For this review, use the dimensioned drawing (mm, ordinates from the lowest corner) and the shaded views. A direction names the side the tool comes from. Give positions to 0.01 mm unless a question says otherwise; leave off trailing zeros. Loops run counter-clockwise (first coordinate to the right, second up) from the corner with the lowest first, then second, coordinate; pieces in that order, holes last. Notation, with made-up numbers: M 71.25,8 L 104.25,8 A14 ccw 104.25,24 Z; hole C -6,13.25 d6. An arc over 180 degrees is marked long. Use a Markdown table: item, result. Add a question column.
(1) For the marked faces 4 and 5, list the 3-axis set-ups (+Z, -Z, +X, -X, +Y, -Y) from which the entire face can be reached by the end or side of a thin tool; tool diameter is ignored.
(2) Draft analysis for pull direction Z (two halves, no side actions). For the marked faces 1, 2 and 3, state which applies: pulls with the +Z half, pulls with the -Z half, needs draft (parallel to the pull), parting line crosses it, or undercut.
(3) Add section B-B, the plane z = 41.1. Give the boundary of the cut face in (x, y), then the cut area to 3 significant figures.
(4) Add section A-A, the plane x = 47. Give the boundary of the cut face in (y, z) (1 decimal).
(5) Insertion check: pin 1 Ø6 at (x, y) = (50.8, 63.5) entering from -Z; pin 2 Ø6 at (x, z) = (29, 6.5) entering from -Y; pin 3 Ø3 at (y, z) = (10.5, 43.5) entering from +X; pin 4 Ø1.9 at (x, z) = (2.5, 29) entering from +Y. Each pin has a flat end and moves straight along its axis. Give the tip position at first contact, or say it passes through.
(6) For probe 1 along X at (y, z) = (63.5, 2.35); probe 2 along Y at (x, z) = (2.25, 15.7); probe 3 along Z at (x, y) = (32, 55), list the stretches that pass through material, from the lowest coordinate up.
(7) Add section C-C, the plane y = 25.4. Give the boundary of the cut face in (x, z) (1 decimal).
(8) Add section D-D, the plane x = 38.1. Give the boundary of the cut face in (y, z) (1 decimal).
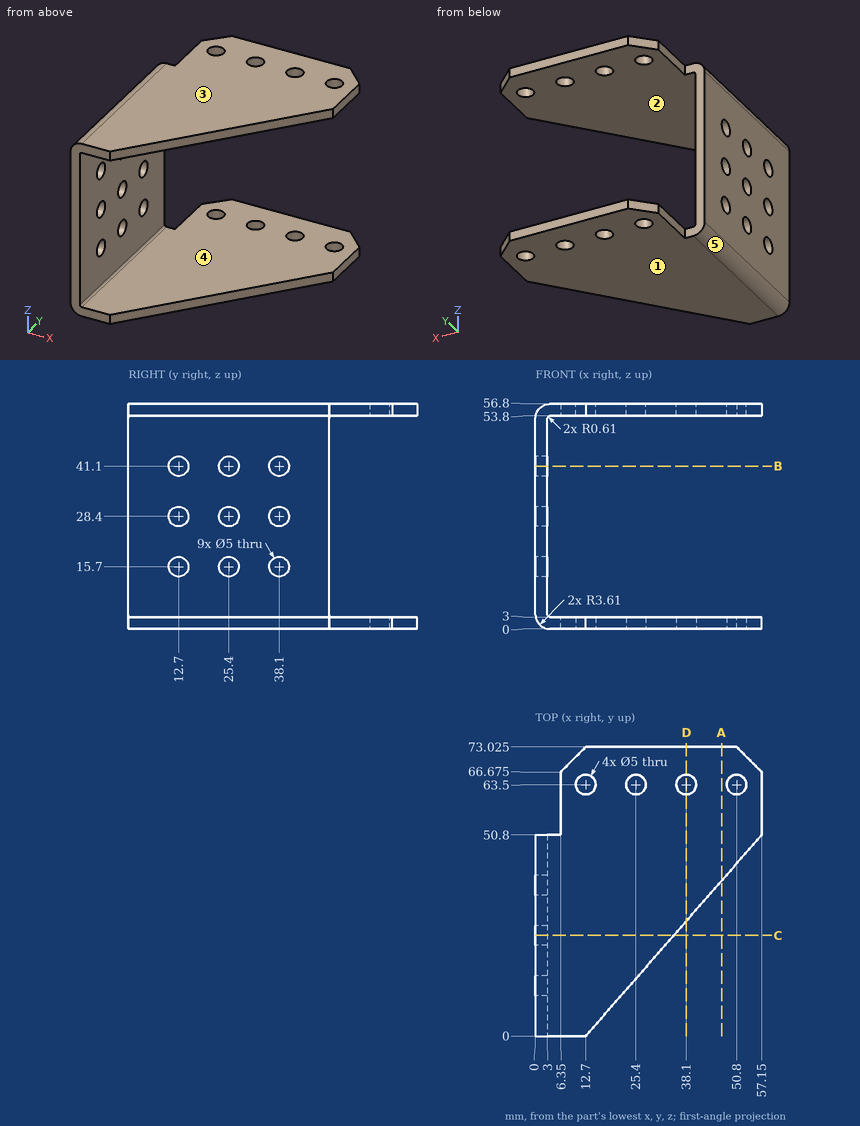
Established:
| question | item | result |
|---|---|---|
| 1 | face 4 | +X, +Y, -Y |
| 1 | face 5 | -Z, -X, +Y, -Y |
| 2 | face 1 | pulls with the -Z half |
| 2 | face 2 | undercut |
| 2 | face 3 | pulls with the +Z half |
| 3 | outline | M 0,0 L 3,0 L 3,10.2 L 0,10.2 Z; M 0,15.2 L 3,15.2 L 3,22.9 L 0,22.9 Z; M 0,27.9 L 3,27.9 L 3,35.6 L 0,35.6 Z; M 0,40.6 L 3,40.6 L 3,50.8 L 0,50.8 Z |
| 3 | area | 107 mm^2 |
| 4 | outline | M 39.2,0 L 73,0 L 73,3 L 39.2,3 Z; M 39.2,53.8 L 73,53.8 L 73,56.8 L 39.2,56.8 Z |
| 5 | pin 1 | z = 0 |
| 5 | pin 2 | through |
| 5 | pin 3 | x = 3 |
| 5 | pin 4 | y = 50.8 |
| 6 | probe 1 | 6.35 to 10.2, 15.2 to 22.9, 27.9 to 35.6, 40.6 to 48.3, 53.3 to 57.15 |
| 6 | probe 2 | 0 to 10.2, 15.2 to 22.9, 27.9 to 35.6, 40.6 to 50.8 |
| 6 | probe 3 | 0 to 3, 53.8 to 56.8 |
| 7 | outline | M 0,3.6 A3.6 ccw 3.6,0 L 34.9,0 L 34.9,3 L 3.6,3 A0.6 cw 3,3.6 L 3,13.2 L 0,13.2 Z; M 0,18.2 L 3,18.2 L 3,25.9 L 0,25.9 Z; M 0,30.9 L 3,30.9 L 3,38.6 L 0,38.6 Z; M 0,43.6 L 3,43.6 L 3,53.2 A0.6 cw 3.6,53.8 L 34.9,53.8 L 34.9,56.8 L 3.6,56.8 A3.6 ccw 0,53.2 Z |
| 8 | outline | M 29,0 L 61,0 L 61,3 L 29,3 Z; M 29,53.8 L 61,53.8 L 61,56.8 L 29,56.8 Z; M 66,0 L 73,0 L 73,3 L 66,3 Z; M 66,53.8 L 73,53.8 L 73,56.8 L 66,56.8 Z |
